from build123d import *

# Parameters (mm, degrees)
F0_R     = 6.35
F0_R_2   = 6.3456189751
F1_DEPTH = 3.175


with BuildPart() as f1:
    # F0 (on Top) → F1 (new body)
    with BuildSketch(Plane.XY):
        with BuildLine():
            Line((94.021920908, 85.0416647869), (89.5317928475, 89.5317928475))
            Line((89.5317928475, 89.5317928475), (85.0416647869, 94.021920908))
            ThreePointArc((85.0416647869, 94.021920908), (80.5515367264, 95.8817928475), (76.0614086659, 94.021920908))
            Line((76.0614086659, 94.021920908), (45.4406379411, 63.4011501833))
            ThreePointArc((45.4406379411, 63.4011501833), (44.5721534378, 62.6753221527), (43.5886052016, 62.1152109764))
            add(Edge.make_bspline(
                [(-62.6577688011, -44.1408912278), (-51.418068027, -19.7331071402), (-28.816494863, 28.7776684856), (19.4337104978, 51.08297888), (43.5886052016, 62.1152109764)],
                knots=[0.0069595994, 0.0069595994, 0.0069595994, 0.0069595994, 0.5011838102, 0.9929298624, 0.9929298624, 0.9929298624, 0.9929298624], degree=3))
            ThreePointArc((-62.6577688011, -44.1408912278), (-63.215282887, -45.1145851352), (-63.9354672331, -45.974954991))
            Line((-63.9354672331, -45.974954991), (-94.5634576344, -76.6029453923))
            ThreePointArc((-94.5634576344, -76.6029453923), (-96.4233295739, -81.0930734528), (-94.5634576344, -85.5832015134))
            Line((-94.5634576344, -85.5832015134), (-90.0733295739, -90.0733295739))
            Line((-90.0733295739, -90.0733295739), (-85.5832015134, -94.5634576344))
            ThreePointArc((-85.5832015134, -94.5634576344), (-81.0930734528, -96.4233295739), (-76.6029453923, -94.5634576344))
            Line((-76.6029453923, -94.5634576344), (-45.974954991, -63.9354672331))
            ThreePointArc((-45.974954991, -63.9354672331), (-45.1145851352, -63.215282887), (-44.1408912278, -62.6577688011))
            add(Edge.make_bspline(
                [(-44.1408912278, -62.6577688011), (-19.7331071402, -51.418068027), (28.7776684856, -28.816494863), (51.08297888, 19.4337104978), (62.1152109764, 43.5886052016)],
                knots=[0.0069595994, 0.0069595994, 0.0069595994, 0.0069595994, 0.5011838102, 0.9929298624, 0.9929298624, 0.9929298624, 0.9929298624], degree=3))
            ThreePointArc((62.1152109764, 43.5886052016), (62.6753221527, 44.5721534378), (63.4011501833, 45.4406379411))
            Line((63.4011501833, 45.4406379411), (94.021920908, 76.0614086659))
            ThreePointArc((94.021920908, 76.0614086659), (95.8817928475, 80.5515367264), (94.021920908, 85.0416647869))
        make_face()
        with Locations((-63.1325612107, -63.1325612107)):
            Circle(F0_R, mode=Mode.SUBTRACT)
        with Locations((-30.3546263688, -30.3546263688)):
            Circle(F0_R, mode=Mode.SUBTRACT)
        Polygon((-31.8156620997, -19.131317284), (-44.4630558556, -29.74374072), (-46.6671745692, -27.1169743245), (-34.0197808133, -16.5045508886), align=None, mode=Mode.SUBTRACT)
        Polygon((13.335, -13.335), (8.255, -13.335), (8.255, -16.51), (-8.255, -16.51), (-8.255, -13.335), (-13.335, -13.335), (-13.335, -8.255), (-16.51, -8.255), (-16.51, 8.255), (-13.335, 8.255), (-13.335, 13.335), (-8.255, 13.335), (-8.255, 16.51), (8.255, 16.51), (8.255, 13.335), (13.335, 13.335), (13.335, 8.255), (16.51, 8.255), (16.51, -8.255), (13.335, -8.255), align=None, mode=Mode.SUBTRACT)
        Polygon((34.0197808133, 16.5045508886), (31.8156620997, 19.131317284), (44.4630558556, 29.74374072), (46.6671745692, 27.1169743245), align=None, mode=Mode.SUBTRACT)
        with Locations((29.8045584932, 29.8045584932)):
            Circle(F0_R_2, mode=Mode.SUBTRACT)
        with Locations((62.5910244843, 62.5910244843)):
            Circle(F0_R, mode=Mode.SUBTRACT)
    extrude(amount=F1_DEPTH)


solid = f1.part
For this review, take the finished solid that the model builds, in its own axes (mm). A direction names the side the tool comes from. Round coordinates to 2 decimals unless told otherwise and drop trailing zeros. Write each loop counter-clockwise with the first axis right and the second up, starting at its lowest first coordinate (ties: lowest second). Pieces come first, ordered by that corner, then holes. Notation, with made-up numbers: (88, 67.5) -> (98, 67.5) arc R23 ccw to (98, 100.5) -> close; hole circle Ø6 at (-18.75, -0.5). An arc over 180 degrees is marked (long way). Put each result on its own line as item: value.
Q1. Consider section B-B on y = 80. State the section outline as (x, z) points (3 decimals), and give its area (3 significant figures).
Determined:
outline: (62.039, 0) -> (95.858, 0) -> (95.858, 3.175) -> (62.039, 3.175) -> close
area: 107 mm^2
Q2. Consider section A-A on z = 2.05. Give the number of separate pieces and of enclosed holes in the cut face, and give its area (3 significant figures).
Determined:
separate pieces: 1
enclosed holes: 7
area: 8,470 mm^2
Q3. Clearance check with flat-ended pins moving along their axes: pin 1 Ø1.6 at (x, z) = (-15, 1) entering from -Y; pin 2 Ø1 at (x, z) = (44, 2.5) entering from +Y; pin 3 Ø1 at (x, z) = (-15, 1) entering from +Y; pin 4 Ø11.5 at (x, y) = (62.59, 62.59) entering from -Z. State where each tip first meets the part, or that it passes through.
Determined:
pin 1: stops at y = -48.98
pin 2: stops at y = 62.63
pin 3: stops at y = 29.38
pin 4: passes through
Q4. The part is to be moulded in two halves that separate along X. For faces 3 (the flat face through (-90.136, -90.01, 1.565)), 4 (the flat face through (40.432, 21.885, 1.565)), 5 (the flat face through (-15, -14, 3.175)), say which applies: released by +X, released by -X, zero draft, split by the parting line, or undercut.
Determined:
face 3: released by -X
face 4: undercut
face 5: zero draft
Q5. To check wall thickness, follow L1, parallel to X at y = -29, z = 0.45; L2, parallel to X at y = -25, z = 2.55; L3, parallel to Y at x = -38, z = 0.8. State the ranges of each line that lie inside material, in increasing order. Write a range as [from, to].
Determined:
L1: x = [-55.58, -45.09], [-43.58, -36.56], [-24.15, 15]
L2: x = [-53.65, -44.14], [-38.81, -33.77], [-26.94, 19.54]
L3: y = [-59.82, -24.32], [-19.84, 2.89]
Q6. Consider section C-C on x = 79. State the section outline as (y, z) points (3 decimals), and give its area (3 significant figures).
Determined:
outline: (61.039, 0) -> (95.689, 0) -> (95.689, 3.175) -> (61.039, 3.175) -> close
area: 110 mm^2
Q7. Machinability: for faces 1 (the flat face through (-79.035, -61.075, 1.565)), 2 (the flat face through (-40.432, -21.885, 1.565)), which of the approach directions +Z, -Z, +X, -X, +Y, -Y give a long, thin tool a straight path to every point of the face, cutting with its end or side? Answer none if there is none.
Determined:
face 1: +Z, -Z, -X, +Y
face 2: +Z, -Z
